The listing builds one solid part. Answer for the finished solid, in the listing's coordinates (mm). Round coordinates to 2 decimals unless told otherwise and drop trailing zeros. Loops run counter-clockwise (first coordinate to the right, second up) from the corner with the lowest first, then second, coordinate; pieces in that order, holes last. Notation, with made-up numbers: (28, 89) -> (45, 89) arc R23 ccw to (45, 100) -> close; hole circle Ø5 at (41, 85.5). An arc over 180 degrees is marked (long way). One line per question, with ' | ' between items.
from build123d import *

# Parameters (mm, degrees)
SKETCH1_R           = 2
SKETCH1_R_2         = 2.162090294
BOSS_EXTRUDE1_DEPTH = 3


with BuildPart() as part:
    # Sketch1 → Boss-Extrude1 (new body)
    with BuildSketch(Plane.XY):
        Polygon((72.5, 104.5), (-72.5, 104.5), (-72.5, 72.5), (-72.5, -72.5), (72.5, -72.5), (72.5, 72.5), align=None)
        with Locations((67, 65.5)):
            Circle(SKETCH1_R, mode=Mode.SUBTRACT)
        with Locations((-35, 65.5)):
            Circle(SKETCH1_R, mode=Mode.SUBTRACT)
        with Locations((-67, 65.5)):
            Circle(SKETCH1_R, mode=Mode.SUBTRACT)
        with Locations((-67, -65.5)):
            Circle(SKETCH1_R, mode=Mode.SUBTRACT)
        with Locations((67, -65.5)):
            Circle(SKETCH1_R, mode=Mode.SUBTRACT)
        with Locations((35, -65.5)):
            Circle(SKETCH1_R, mode=Mode.SUBTRACT)
        with Locations((21, -66)):
            Circle(SKETCH1_R_2, mode=Mode.SUBTRACT)
        with Locations((-21, -66)):
            Circle(SKETCH1_R_2, mode=Mode.SUBTRACT)
        with Locations((-9, -42.5)):
            Circle(SKETCH1_R, mode=Mode.SUBTRACT)
        with Locations((9, -66.5)):
            Circle(SKETCH1_R, mode=Mode.SUBTRACT)
        with Locations((9, 66.5)):
            Circle(SKETCH1_R, mode=Mode.SUBTRACT)
        with Locations((-9, 66.5)):
            Circle(SKETCH1_R, mode=Mode.SUBTRACT)
        with Locations((-9, 42.5)):
            Circle(SKETCH1_R, mode=Mode.SUBTRACT)
        with Locations((9, 42.5)):
            Circle(SKETCH1_R, mode=Mode.SUBTRACT)
        with Locations((-9, -66.5)):
            Circle(SKETCH1_R, mode=Mode.SUBTRACT)
        with Locations((9, -42.5)):
            Circle(SKETCH1_R, mode=Mode.SUBTRACT)
        with Locations((-35, -65.5)):
            Circle(SKETCH1_R, mode=Mode.SUBTRACT)
        with Locations((35, 65.5)):
            Circle(SKETCH1_R, mode=Mode.SUBTRACT)
    extrude(amount=BOSS_EXTRUDE1_DEPTH)


solid = part.part
Q1. A cutting plane is placed at A-A on x = 35. Give the vertices of the cut face in (y, z), plus the area to 3 significant figures.
Numbers:
outline: (-72.5, 0) -> (-67.5, 0) -> (-67.5, 3) -> (-72.5, 3) -> close; (-63.5, 0) -> (63.5, 0) -> (63.5, 3) -> (-63.5, 3) -> close; (67.5, 0) -> (104.5, 0) -> (104.5, 3) -> (67.5, 3) -> close | area: 507 mm^2
Q2. A cutting plane is placed at C-C on x = -9. Give the vertices of the cut face in (y, z).
Numbers:
outline: (-72.5, 0) -> (-68.5, 0) -> (-68.5, 3) -> (-72.5, 3) -> close; (-64.5, 0) -> (-44.5, 0) -> (-44.5, 3) -> (-64.5, 3) -> close; (-40.5, 0) -> (40.5, 0) -> (40.5, 3) -> (-40.5, 3) -> close; (44.5, 0) -> (64.5, 0) -> (64.5, 3) -> (44.5, 3) -> close; (68.5, 0) -> (104.5, 0) -> (104.5, 3) -> (68.5, 3) -> close
Q3. A cutting plane is placed at B-B on y = -42.5. Give the vertices of the cut face in (x, z).
Numbers:
outline: (-72.5, 0) -> (-11, 0) -> (-11, 3) -> (-72.5, 3) -> close; (-7, 0) -> (7, 0) -> (7, 3) -> (-7, 3) -> close; (11, 0) -> (72.5, 0) -> (72.5, 3) -> (11, 3) -> close
Q4. For a pull along X with two mould halves and no side action, classify faces 1 (the face through (-9.434, -44.452, 1.479)), 2 (the face through (-1, 17, 0)) as pulls with the +X half, pulls with the -X half, needs draft (parallel to the pull), parting line crosses it, or undercut.
Numbers:
face 1: undercut | face 2: needs draft
Q5. Given pin 1 Ø7 at (x, y) = (21, -66) entering from +Z, flat-ended and moving along its own axis, determine where the tip first touches the part or whether it passes through.
Numbers:
pin 1: z = 3
Q6. Find the intervals of material crossed by line 1 (Y direction, x = -35, z = 1.9); line 2 (Y direction, x = -9, z = 0.8); line 3 (X direction, y = 68, z = 2.65), in increasing order. Write a range as from..to.
Numbers:
line 1: -72.5..-67.5, -63.5..63.5, 67.5..104.5 | line 2: -72.5..-68.5, -64.5..-44.5, -40.5..40.5, 44.5..64.5, 68.5..104.5 | line 3: -72.5..-10.32, -7.68..7.68, 10.32..72.5
